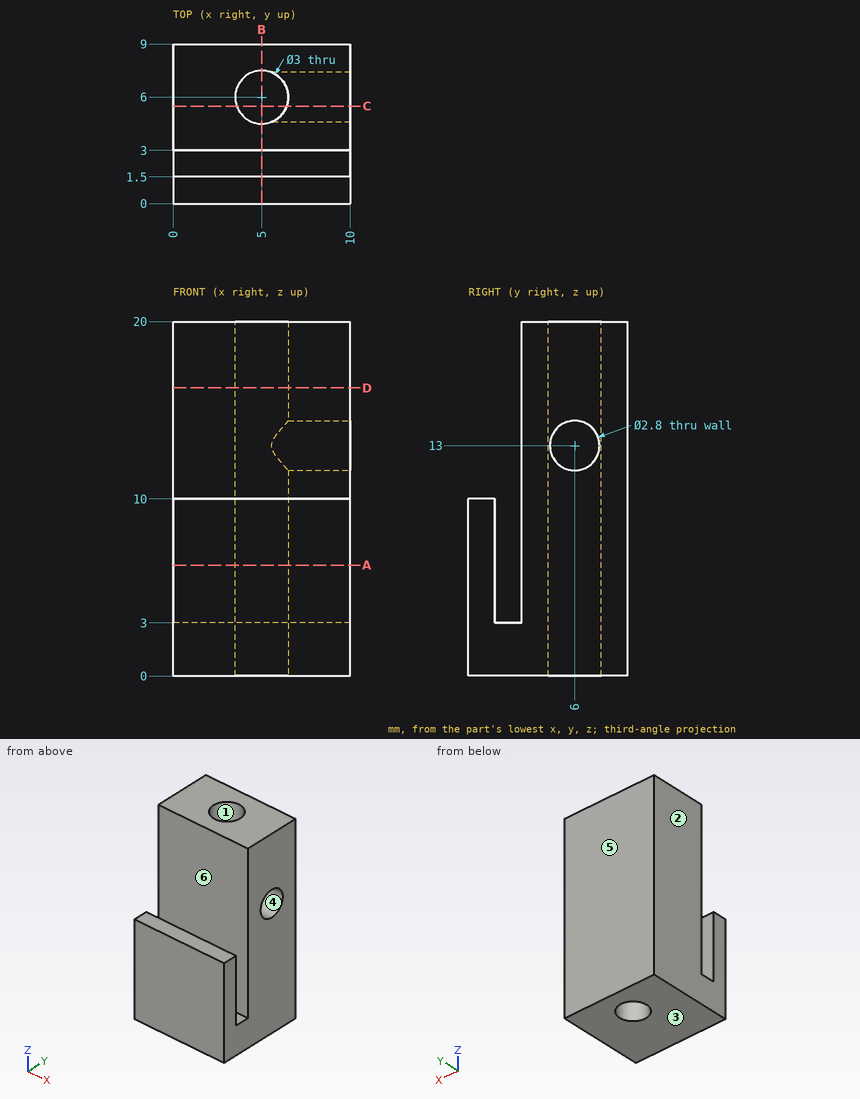
Design review of the part shown in the three views and the two pictorial views. Dimensions are in mm from the part's minimum x, y and z. A direction names the side the tool comes from. Give positions to 0.01 mm unless a question says otherwise; leave off trailing zeros. Loops run counter-clockwise (first coordinate to the right, second up) from the corner with the lowest first, then second, coordinate; pieces in that order, holes last. Notation, with made-up numbers: (67, 69.5) - (87, 69.5) arc R31 ccw to (87, 93.5) - close; hole circle Ø4 at (50, 73.5). An arc over 180 degrees is marked (long way). Answer as a JSON object with one key per item and string values.
Q1. Add section D-D on z = 16.25. State the section outline as (x, y) points.
Worked out:
{"outline": "(0, 3) - (10, 3) - (10, 9) - (0, 9) - close; hole circle Ø3 at (5, 6)"}
Q2. Mouldability with a two-part tool opening along X and no side actions: class the marked faces 1, 2 and 3 as +X half, -X half, draft (parallel to the pull), parting line (faces both ways), or undercut.
Worked out:
{"face 1": "undercut", "face 2": "-X half", "face 3": "draft"}
Q3. To check wall thickness, follow line 1 along Z through (x, y) = (7.7, 6); line 2 along Y through (x, z) = (1.5, 7.75); line 3 along Y through (x, z) = (6.25, 5). State the ranges of each line that lie inside material, in increasing order.
Worked out:
{"line 1": "z = 0 to 11.6, 14.4 to 20", "line 2": "y = 0 to 1.5, 3 to 9", "line 3": "y = 0 to 1.5, 3 to 5.17, 6.83 to 9"}
Q4. For the marked faces 4, 5 and 6, list the 3-axis set-ups (+Z, -Z, +X, -X, +Y, -Y) from which the entire face can be reached by the end or side of a thin tool; tool diameter is ignored.
Worked out:
{"face 4": "+X", "face 5": "+Z, -Z, +X, -X, +Y", "face 6": "+Z, +X, -X"}
Q5. Add section B-B on x = 5. State the section outline as (y, z) points.
Worked out:
{"outline": "(0, 0) - (4.5, 0) - (4.5, 20) - (3, 20) - (3, 3) - (1.5, 3) - (1.5, 10) - (0, 10) - close; (7.5, 0) - (9, 0) - (9, 20) - (7.5, 20) - close"}
Q6. Add section A-A on z = 6.25. State the section outline as (x, y) points, plus the area to 3 significant figures.
Worked out:
{"outline": "(0, 0) - (10, 0) - (10, 1.5) - (0, 1.5) - close; (0, 3) - (10, 3) - (10, 9) - (0, 9) - close; hole circle Ø3 at (5, 6)", "area": "67.9 mm^2"}
Q7. Add section C-C on y = 5.5. State the section outline as (x, z) points, plus the area to 3 significant figures.
Worked out:
{"outline": "(0, 0) - (3.59, 0) - (3.59, 20) - (0, 20) - close; (6.41, 0) - (10, 0) - (10, 11.69) - (6.41, 11.69) - close; (6.41, 14.31) - (10, 14.31) - (10, 20) - (6.41, 20) - close", "area": "134 mm^2"}
